```python
from build123d import *

# Parameters (mm, degrees)
SKETCH1_W               = 30.988
SKETCH1_H               = 34.925
BOSS_EXTRUDE1_DEPTH     = 1.524
SKETCH2_R               = 8.4455
CUT_EXTRUDE1_DEPTH      = 24.39498917
CUT_EXTRUDE2_DEPTH      = 24.39498917
SKETCH4_W               = 6.35
SKETCH4_H               = 1.524
BOSS_EXTRUDE2_DEPTH     = 1.524
SKETCH4_3_R             = 0.79375
CUT_EXTRUDE3_DEPTH      = 25.553488433
MIRROR4_COPY_1_DEPTH    = 24.39498917
MIRROR4_COPY_2_SKETCH_W = 6.35
MIRROR4_COPY_2_SKETCH_H = 1.524
MIRROR4_COPY_2_DEPTH    = 1.524
MIRROR4_COPY_3_SKETCH_R = 0.79375
MIRROR4_COPY_3_DEPTH    = 25.553488433


with BuildPart() as part:
    # Sketch1 → Boss-Extrude1 (new body)
    with BuildSketch(Plane.XY):
        Rectangle(SKETCH1_W, SKETCH1_H)
    extrude(amount=BOSS_EXTRUDE1_DEPTH)

    # Sketch2 → Cut-Extrude1 (cut, through all)
    with BuildSketch(Plane.XY.offset(1.524)):
        Circle(SKETCH2_R)
        with BuildLine():
            ThreePointArc((1.4605, -8.31825763), (0, -8.4455), (-1.4605, -8.31825763))
            Line((-1.4605, -8.31825763), (-1.4605, -11.0617))
            ThreePointArc((-1.4605, -11.0617), (-1.222436392, -11.636436392), (-0.6477, -11.8745))
            Line((-0.6477, -11.8745), (0.6477, -11.8745))
            ThreePointArc((0.6477, -11.8745), (1.222436392, -11.636436392), (1.4605, -11.0617))
            Line((1.4605, -11.0617), (1.4605, -8.31825763))
        make_face()
    extrude(amount=-CUT_EXTRUDE1_DEPTH, mode=Mode.SUBTRACT)

    # Sketch3 → Cut-Extrude2 (cut, through all)
    with BuildSketch(Plane.XY.offset(1.524)):
        with BuildLine():
            Line((15.494, 13.1445), (13.843, 13.1445))
            ThreePointArc((13.843, 13.1445), (12.954, 14.0335), (13.843, 14.9225))
            Line((13.843, 14.9225), (15.494, 14.9225))
            ThreePointArc((15.494, 14.9225), (16.383, 14.0335), (15.494, 13.1445))
        make_face()
    cut_extrude2 = extrude(amount=-CUT_EXTRUDE2_DEPTH, mode=Mode.SUBTRACT)

    # Sketch4 → Boss-Extrude2 (add)
    with BuildSketch(Plane.XY.offset(1.524)):
        with Locations((8.255, 18.2245)):
            Rectangle(SKETCH4_W, SKETCH4_H)
    boss_extrude2 = extrude(amount=-BOSS_EXTRUDE2_DEPTH)

    # Sketch4<3> → Cut-Extrude3 (cut, through all)
    with BuildSketch(Plane.XY.offset(1.524)):
        with Locations((4.28625, 17.4625)):
            Circle(SKETCH4_3_R)
    cut_extrude3 = extrude(amount=-CUT_EXTRUDE3_DEPTH, mode=Mode.SUBTRACT)

    # Mirror3: Cut-Extrude2, Boss-Extrude2, Cut-Extrude3 across plane
    add(cut_extrude2.mirror(Plane.ZX), mode=Mode.SUBTRACT)
    add(boss_extrude2.mirror(Plane.ZX))
    add(cut_extrude3.mirror(Plane.ZX), mode=Mode.SUBTRACT)

    # Mirror4: Cut-Extrude2, Boss-Extrude2, Cut-Extrude3 across plane
    add(cut_extrude2.mirror(Plane(origin=(0, 0, 0), x_dir=(0, 0, 1), z_dir=(1, 0, 0))), mode=Mode.SUBTRACT)
    add(boss_extrude2.mirror(Plane(origin=(0, 0, 0), x_dir=(0, 0, 1), z_dir=(1, 0, 0))))
    add(cut_extrude3.mirror(Plane(origin=(0, 0, 0), x_dir=(0, 0, 1), z_dir=(1, 0, 0))), mode=Mode.SUBTRACT)

    # Mirror4 copy 1 sketch → Mirror4 copy 1 (cut, through all)
    with BuildSketch(Plane(origin=(0, 0, 1.524), x_dir=(-1, 0, 0), z_dir=(0, 0, 1))):
        with BuildLine():
            Line((15.494, 13.1445), (13.843, 13.1445))
            ThreePointArc((13.843, 13.1445), (12.954, 14.0335), (13.843, 14.9225))
            Line((13.843, 14.9225), (15.494, 14.9225))
            ThreePointArc((15.494, 14.9225), (16.383, 14.0335), (15.494, 13.1445))
        make_face()
    extrude(amount=-MIRROR4_COPY_1_DEPTH, mode=Mode.SUBTRACT)

    # Mirror4 copy 2 sketch → Mirror4 copy 2 (add)
    with BuildSketch(Plane(origin=(0, 0, 1.524), x_dir=(-1, 0, 0), z_dir=(0, 0, 1))):
        with Locations((8.255, 18.2245)):
            Rectangle(MIRROR4_COPY_2_SKETCH_W, MIRROR4_COPY_2_SKETCH_H)
    extrude(amount=-MIRROR4_COPY_2_DEPTH)

    # Mirror4 copy 3 sketch → Mirror4 copy 3 (cut, through all)
    with BuildSketch(Plane(origin=(0, 0, 1.524), x_dir=(-1, 0, 0), z_dir=(0, 0, 1))):
        with Locations((4.28625, 17.4625)):
            Circle(MIRROR4_COPY_3_SKETCH_R)
    extrude(amount=-MIRROR4_COPY_3_DEPTH, mode=Mode.SUBTRACT)


solid = part.part
```
Check sheet for the modelled part. Datum: model origin and axes. Units: mm. A direction names the side the tool comes from. Give positions to 0.01 mm unless a question says otherwise; leave off trailing zeros. Write each loop counter-clockwise with the first axis right and the second up, starting at its lowest first coordinate (ties: lowest second). Pieces come first, ordered by that corner, then holes. Notation, with made-up numbers: (3, 33.25) - (44, 33.25) arc R24 cw to (44, 69.25) - close; hole circle Ø10 at (1, -40). An arc over 180 degrees is marked (long way). Answer as a JSON object with one key per item and string values. Group by question number.
1) Release check for a two-part mould opening along X. For faces 4 (the face through (4.27, 16.67, 0.77)), 5 (the face through (-12.954, -14.014, 0.773)), 6 (the face through (15, 14.922, 1)) record: pulls with the +X half, pulls with the -X half, needs draft (parallel to the pull), parting line crosses it, or undercut.
2) Sectioned sample at B-B (x = -2.5). Record the cut outline in (y, z).
3) Depth check by flat-ended pin: P1, Ø0.8, axis at x = 0, z = 0.5, coming from the -Y side; P2, Ø0.6, axis at x = 0, z = 0.5, coming from the +Y side; P3, Ø0.5, axis at y = -18, z = 0.5, coming from the +X side. Enter the tip coordinate at first touch or a pass-through.
4) Thickness scan on probe 1 along X at (y, z) = (0, 0.55); probe 2 along X at (y, z) = (17.5, 0.1); probe 3 along Y at (x, z) = (0, 0.85). Record the ranges inside material, lowest first. Write a range as from..to.
5) Access from +Z, -Z, +X, -X, +Y, -Y to the whole of each face (thin tool, end or side, straight path). Record for faces 1 (the face through (15, -13.144, 1)), 2 (the face through (11.43, -18, 1)), 3 (the face through (-13, 17.462, 1)).
6) Sectioned sample at A-A (y = 0). Record the cut outline in (x, z), then the cut area to 3 significant figures.
Geometry results:
{
 "1": {"face 4": "undercut", "face 5": "pulls with the -X half", "face 6": "needs draft"},
 "2": {"outline": "(-17.46, 0) - (-8.07, 0) - (-8.07, 1.52) - (-17.46, 1.52) - close; (8.07, 0) - (17.46, 0) - (17.46, 1.52) - (8.07, 1.52) - close"},
 "3": {"P1": "stops at y = -17.46", "P2": "stops at y = 17.46", "P3": "stops at x = 11.43"},
 "4": {"probe 1": "x = -15.49..-8.45, 8.45..15.49", "probe 2": "x = -11.43..-5.08, 5.08..11.43", "probe 3": "y = -17.46..-11.87, 8.45..17.46"},
 "5": {"face 1": "+Z, -Z, +X", "face 2": "+Z, -Z, +X, -Y", "face 3": "+Z, -Z, -X, +Y"},
 "6": {"outline": "(-15.49, 0) - (-8.45, 0) - (-8.45, 1.52) - (-15.49, 1.52) - close; (8.45, 0) - (15.49, 0) - (15.49, 1.52) - (8.45, 1.52) - close", "area": "21.5 mm^2"}
}
